Verification items for the finished model (mm, model axes). A direction names the side the tool comes from. Coordinates: 2 decimals unless noted, no trailing zeros. Loops run counter-clockwise (first coordinate to the right, second up) from the corner with the lowest first, then second, coordinate; pieces in that order, holes last. Notation, with made-up numbers: (-38.75, -33.5) -> (-24.75, -33.5) arc R35 cw to (-24.75, 5.5) -> close; hole circle Ø1 at (79.5, 82.25). An arc over 180 degrees is marked (long way). Use CSV: the item, a comma, the result in double quotes. Start each with the question number.
```python
from build123d import *

# Parameters (mm, degrees)
SKETCH1_R           = 30
BOSS_EXTRUDE3_DEPTH = 6
BOSS_EXTRUDE2_DEPTH = 6
CIRPATTERN3_COUNT   = 22
SKETCH5_R           = 9.75
BOSS_EXTRUDE4_DEPTH = 10.7
SKETCH6_R           = 3
CUT_EXTRUDE1_DEPTH  = 49.191740155


with BuildPart() as part:
    # Sketch1 → Boss-Extrude3 (new body)
    with BuildSketch(Plane(origin=(0, 0, 0), x_dir=(1, 0, 0), z_dir=(0, 1, 0))):
        with Locations(Location((0, 0, 0), (0, 0, 270))):
            Circle(SKETCH1_R)
    extrude(amount=BOSS_EXTRUDE3_DEPTH)

    # Sketch2 → Boss-Extrude2 (add)
    with BuildSketch(Plane(origin=(0, 6, 0), x_dir=(1, 0, 0), z_dir=(0, 1, 0))):
        Polygon((0, 32), (1.8, 32), (3.407695155, 26), (0, 26), (-3.407695155, 26), (-1.8, 32), align=None)
    boss_extrude2 = extrude(amount=-BOSS_EXTRUDE2_DEPTH)

    # CirPattern3: Boss-Extrude2 ×22 about axis
    cirpattern3_axis = Axis((0, 0, 0), (0, 1, 0))
    for i in range(1, CIRPATTERN3_COUNT):
        add(boss_extrude2.rotate(cirpattern3_axis, i * 360 / CIRPATTERN3_COUNT))

    # Sketch5 → Boss-Extrude4 (add)
    with BuildSketch(Plane(origin=(0, 6, 0), x_dir=(1, 0, 0), z_dir=(0, 1, 0))):
        with Locations(Location((0, 0, 0), (0, 0, 270))):
            Circle(SKETCH5_R)
    extrude(amount=BOSS_EXTRUDE4_DEPTH)

    # Sketch6 → Cut-Extrude1 (cut, through all)
    with BuildSketch(Plane(origin=(0, 16.7, 0), x_dir=(1, 0, 0), z_dir=(0, 1, 0))):
        with Locations(Location((0, 0, 0), (0, 0, 270))):
            Circle(SKETCH6_R)
    extrude(amount=-CUT_EXTRUDE1_DEPTH, mode=Mode.SUBTRACT)


solid = part.part
```
1. Cross-section at B-B, the plane x = 0. Record the boundary of the cut face in (y, z), plus the area to 3 significant figures.
2. Scan lines: line 1 (X direction, y = 6.75, z = 0); line 2 (X direction, y = 5, z = 0); line 3 (Y direction, x = -28, z = 6). Record each from-to range of solid material in increasing order.
3. Set-up check for faces 1 (the flat face through (-22.044, 3.042, -21.849)), 2 (the cylindrical face through (19.67, 2.96, -22.65)), 3 (the flat face through (30.948, 3.042, -2.352)), 4 (the flat face through (-24.764, 3.042, 18.711)): record each of +Z, -Z, +X, -X, +Y, -Y from which the full face is reachable in a straight line by a thin tool's end or side.
4. Cross-section at A-A, the plane z = 0. Record the boundary of the cut face in (x, y), plus the area to 3 significant figures.
5. Depth check by flat-ended pin: pin 1 (4 mm diameter, centred on x = 20.5, y = 2, fed in from -Z); pin 2 (5 mm diameter, centred on x = 2, z = -17, fed in from +Y); pin 3 (3 mm diameter, centred on x = -2, y = 13, fed in from -Z). Enter the tip coordinate at first touch or a pass-through.
6. Release check for a two-part mould opening along X. For faces 5 (the flat face through (-29.01, 3.04, -10.96)), 6 (the flat face through (0, 3, -32)), 7 (the flat face through (17.322, 3.042, -26.906)), 8 (the cylindrical face through (-4.3, 2.96, 29.69)) record: released by +X, released by -X, zero draft, split by the parting line, or undercut.
7. Cross-section at C-C, the plane y = 13.75. Record the boundary of the cut face in (x, z), plus the area to 3 significant figures.
Solution:
1,outline,"(0, -32) -> (6, -32) -> (6, -9.75) -> (16.7, -9.75) -> (16.7, -3) -> (0, -3) -> close; (0, 3) -> (16.7, 3) -> (16.7, 9.75) -> (6, 9.75) -> (6, 32) -> (0, 32) -> close"
1,area,"492 mm2"
2,line 1,"x = -9.75 to -3, 3 to 9.75"
2,line 2,"x = -30 to -3, 3 to 30"
2,line 3,"y = 0 to 6"
3,face 1,"-Z, +Y, -Y"
3,face 2,"+Y, -Y"
3,face 3,"+X, +Y, -Y"
3,face 4,"-X, +Y, -Y"
4,outline,"(-30, 0) -> (-3, 0) -> (-3, 16.7) -> (-9.75, 16.7) -> (-9.75, 6) -> (-30, 6) -> close; (3, 0) -> (30, 0) -> (30, 6) -> (9.75, 6) -> (9.75, 16.7) -> (3, 16.7) -> close"
4,area,"468 mm2"
5,pin 1,"stops at z = -26.15"
5,pin 2,"stops at y = 6"
5,pin 3,"stops at z = -9.74"
6,face 5,"released by -X"
6,face 6,"zero draft"
6,face 7,"released by +X"
6,face 8,"undercut"
7,outline,"circle Ø19.5 at (0, 0); hole circle Ø6 at (0, 0)"
7,area,"270 mm2"
